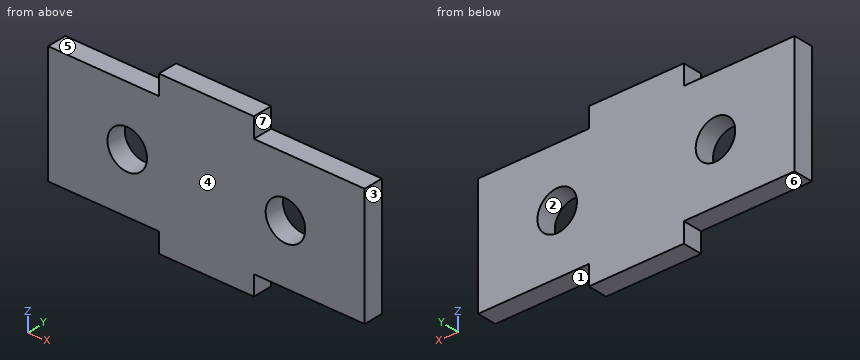
```python
from build123d import *

# Parameters (mm, degrees)
F0_R     = 3.175
F1_DEPTH = 3.175


with BuildPart() as f1:
    # F0 (on Front) → F1 (new body)
    with BuildSketch(Plane.XZ):
        Polygon((-7.62, -12.695253), (7.62, -12.695253), (7.62, -9.525), (25.4, -9.525), (25.4, -6.35), (25.4, 6.357342), (25.4, 9.525), (7.62, 9.525), (7.62, 12.7), (-7.62, 12.7), (-7.62, 9.525), (-25.4, 9.525), (-25.4, 6.355764), (-25.4, -6.35), (-25.4, -9.525), (-7.62, -9.525), align=None)
        with Locations((-12.7, 0)):
            Circle(F0_R, mode=Mode.SUBTRACT)
        with Locations((12.7, 0)):
            Circle(F0_R, mode=Mode.SUBTRACT)
    extrude(amount=F1_DEPTH)


solid = f1.part
```
Model file for the job. Use its own axes, mm. Face numbers are marked on the shaded views. A direction names the side the tool comes from. Coordinates: 2 decimals unless noted, no trailing zeros. Order: outer loops, then holes, each group sorted by start corner. A loop starts at its lowest first (then second) coordinate and runs counter-clockwise, first axis right, second up. Notation, with made-up numbers: (-9.75, -26) -> (3.25, -26) arc R22 ccw to (3.25, -2) -> close; hole circle Ø9 at (-12, -6.75). An arc over 180 degrees is marked (long way). Return JSON: item names as keys, results as strings.
Item 1: Mould opens along Z. For the marked faces 1, 2 and 3 say: pulls with the +Z half, pulls with the -Z half, needs draft (parallel to the pull), parting line crosses it, or undercut.
Model answer:
{"face 1": "pulls with the -Z half", "face 2": "undercut", "face 3": "needs draft"}
Item 2: Wall check: line 1 along Z through (x, y) = (12.7, -1.5) (3 decimals); line 2 along X through (y, z) = (-1.75, 2.25); line 3 along X through (y, z) = (-1.5, 0.5). Give the ranges that are in metal, low to high. Write a range as from..to.
Model answer:
{"line 1": "z = -9.525..-3.175, 3.175..9.525", "line 2": "x = -25.4..-14.94, -10.46..10.46, 14.94..25.4", "line 3": "x = -25.4..-15.84, -9.56..9.56, 15.84..25.4"}
Item 3: 3-axis set-ups, long thin cutter, end or side, ignore diameter. For the marked faces 4, 5, 6 and 7: which of +Z, -Z, +X, -X, +Y, -Y reach the whole face in a straight line?
Model answer:
{"face 4": "+Z, -Z, +X, -X, -Y", "face 5": "+Z, -X, +Y, -Y", "face 6": "-Z, -X, +Y, -Y", "face 7": "+Z, +X, +Y, -Y"}
Item 4: Pin check, flat tips, straight feed: P1, Ø1.6, axis at y = -1.5, z = 11, coming from the +X side; P2, Ø1, axis at y = -1.5, z = 11, coming from the -X side; P3, Ø1.6, axis at x = -19.5, y = -1, coming from the -Z side (3 decimals). Stop position of each tip, or through.
Model answer:
{"P1": "stops at x = 7.62", "P2": "stops at x = -7.62", "P3": "stops at z = -9.525"}
Item 5: Slice it at B-B (z = 0). Write the cut outline in (x, y) (3 decimals).
Model answer:
{"outline": "(-25.4, -3.175) -> (-15.875, -3.175) -> (-15.875, 0) -> (-25.4, 0) -> close; (-9.525, -3.175) -> (9.525, -3.175) -> (9.525, 0) -> (-9.525, 0) -> close; (15.875, -3.175) -> (25.4, -3.175) -> (25.4, 0) -> (15.875, 0) -> close"}
Item 6: Slice it at D-D (z = 10.5). Write the cut outline in (x, y) (3 decimals), then the cut area to 3 significant figures.
Model answer:
{"outline": "(-7.62, -3.175) -> (7.62, -3.175) -> (7.62, 0) -> (-7.62, 0) -> close", "area": "48.4 mm²"}
Item 7: Slice it at A-A (x = 12.7). Write the cut outline in (y, z) (3 decimals).
Model answer:
{"outline": "(-3.175, -9.525) -> (0, -9.525) -> (0, -3.175) -> (-3.175, -3.175) -> close; (-3.175, 3.175) -> (0, 3.175) -> (0, 9.525) -> (-3.175, 9.525) -> close"}
Item 8: Slice it at C-C (y = -1.45). Write the cut outline in (x, z) (3 decimals), then the cut area to 3 significant figures.
Model answer:
{"outline": "(-25.4, -9.525) -> (-7.62, -9.525) -> (-7.62, -12.695) -> (7.62, -12.695) -> (7.62, -9.525) -> (25.4, -9.525) -> (25.4, 9.525) -> (7.62, 9.525) -> (7.62, 12.7) -> (-7.62, 12.7) -> (-7.62, 9.525) -> (-25.4, 9.525) -> close; hole circle Ø6.35 at (-12.7, 0); hole circle Ø6.35 at (12.7, 0)", "area": "1,000 mm²"}
